Could you check a few things on this drawing? It's one solid part, dimensions in mm from its lowest x, y, z. A direction names the side the tool comes from. Coordinates: 2 decimals unless noted, no trailing zeros. Write each loop counter-clockwise with the first axis right and the second up, starting at its lowest first coordinate (ties: lowest second). Pieces come first, ordered by that corner, then holes.
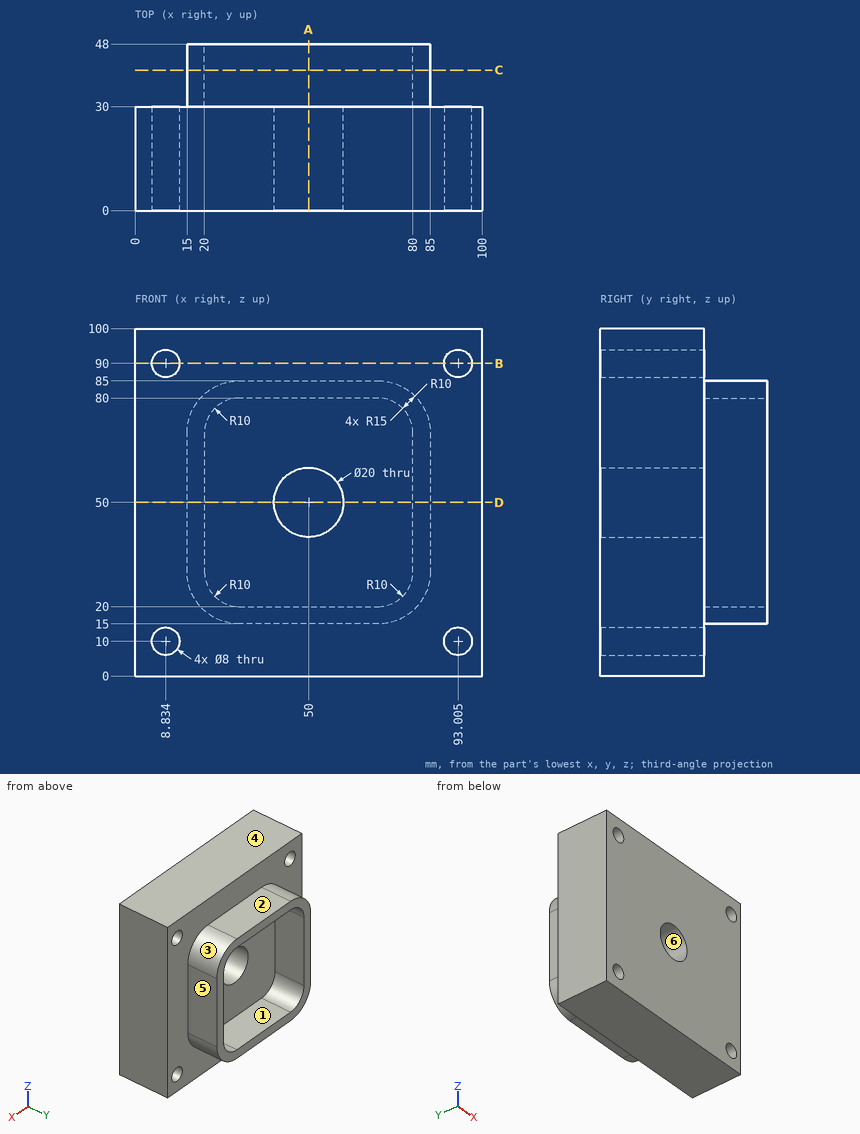
1) Will these pins go through, and if not, where does the flat tip stop? pin 1 (8 mm diameter, centred on x = 48, z = 40.5, fed in from +Y); pin 2 (5.5 mm diameter, centred on x = 46.5, y = 35, fed in from +Z); pin 3 (9 mm diameter, centred on x = 58, y = 35, fed in from -Z).
Values follow:
pin 1: stops at y = 30
pin 2: stops at z = 85
pin 3: stops at z = 15
2) On a 3-axis mill with a long thin cutter (end or side, diameter ignored), from which of +Z, -Z, +X, -X, +Y, -Y can I reach the whole of each face in a straight line? I mean the marked faces 1, 2 and 3. Say none if no direction works.
Values follow:
face 1: +Y
face 2: +Z, +X, -X, +Y
face 3: +Z, +X, +Y
3) We'd pull the mould along Z, two halves only. Please class the marked faces 4, 5 and 6: pulls with the +Z half, pulls with the -Z half, needs draft (parallel to the pull), parting line crosses it, or undercut.
Values follow:
face 4: pulls with the +Z half
face 5: needs draft
face 6: undercut
4) Imagine slicing it at A-A on x = 50. Please give me the cut outline in (y, z), then the cut area to 3 significant figures.
Values follow:
outline: (0, 0) - (30, 0) - (30, 15) - (48, 15) - (48, 20) - (30, 20) - (30, 40) - (0, 40) - close; (0, 60) - (30, 60) - (30, 80) - (48, 80) - (48, 85) - (30, 85) - (30, 100) - (0, 100) - close
area: 2,580 mm2
5) Imagine slicing it at C-C on y = 40.5. Please give me the cut outline in (x, z).
Values follow:
outline: (15, 30) arc R15 ccw to (30, 15) - (70, 15) arc R15 ccw to (85, 30) - (85, 70) arc R15 ccw to (70, 85) - (30, 85) arc R15 ccw to (15, 70) - close; hole (20, 30) arc R10 ccw to (30, 20) - (70, 20) arc R10 ccw to (80, 30) - (80, 70) arc R10 ccw to (70, 80) - (30, 80) arc R10 ccw to (20, 70) - close
6) Imagine slicing it at D-D on z = 50. Please give me the cut outline in (x, y).
Values follow:
outline: (0, 0) - (40, 0) - (40, 30) - (20, 30) - (20, 48) - (15, 48) - (15, 30) - (0, 30) - close; (60, 0) - (100, 0) - (100, 30) - (85, 30) - (85, 48) - (80, 48) - (80, 30) - (60, 30) - close
7) I need wall thicknesses on probe 1 along Z at (x, y) = (50, 12); probe 2 along Z at (x, y) = (69, 44); probe 3 along Y at (x, z) = (85, 79.5). Which ranges of each line are inside material? Lowest first, please.
Values follow:
probe 1: z = 0 to 40, 60 to 100
probe 2: z = 15 to 20, 80 to 85
probe 3: y = 0 to 30
8) Imagine slicing it at B-B on z = 90. Please give me the cut outline in (x, y) (1 decimal), then the cut area to 3 significant figures.
Values follow:
outline: (0, 0) - (4.8, 0) - (4.8, 30) - (0, 30) - close; (12.8, 0) - (89, 0) - (89, 30) - (12.8, 30) - close; (97, 0) - (100, 0) - (100, 30) - (97, 30) - close
area: 2,520 mm2
